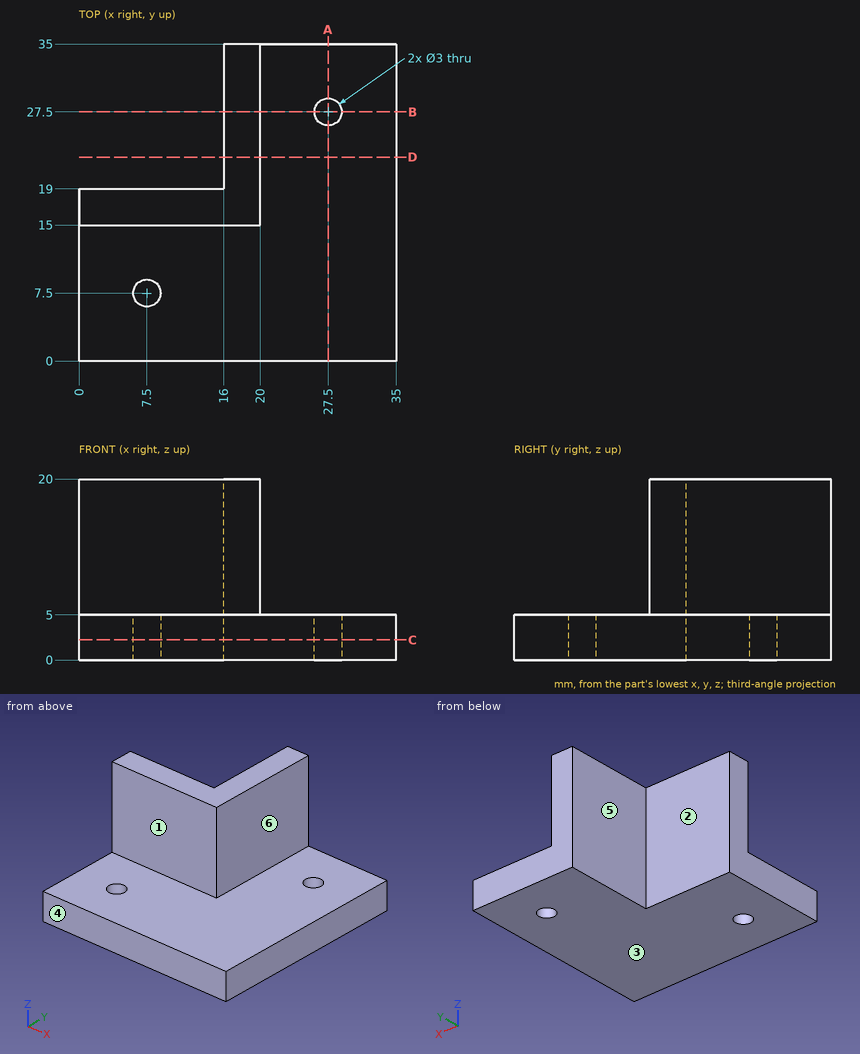
Study the drawing (mm; zero at the part's minimum x, y, z) and answer. A direction names the side the tool comes from. Coordinates: 2 decimals unless noted, no trailing zeros. Write each loop counter-clockwise with the first axis right and the second up, starting at its lowest first coordinate (ties: lowest second). Pieces come first, ordered by that corner, then holes. Notation, with made-up numbers: (85, 61.25) - (107, 61.25) arc R9 cw to (107, 78.25) - close; hole circle Ø11 at (32, 5). An arc over 180 degrees is marked (long way). One line per item, written item: value.
1) Find section A-A (x = 27.5). Give the vertices of the cut face in (y, z), and give its area (3 significant figures).
Geometry check:
outline: (0, 0) - (26, 0) - (26, 5) - (0, 5) - close; (29, 0) - (35, 0) - (35, 5) - (29, 5) - close
area: 160 mm2
2) Each of these flat-tipped pins is pushed along its axis until it touches: pin 1 Ø12 at (y, z) = (28.5, 16) entering from +X; pin 2 Ø5 at (y, z) = (25.5, 6.5) entering from -X; pin 3 Ø1.5 at (x, y) = (22.5, 15.5) entering from +Z. Where does it stop, or does it pass through?
Geometry check:
pin 1: stops at x = 20
pin 2: stops at x = 16
pin 3: stops at z = 5
3) A tool of negligible diameter and unlimited length cuts with its end or side. For the marked faces 4, 5 and 6, from which of +Z, -Z, +X, -X, +Y, -Y can it reach the whole face along a straight path? Write none if from no direction.
Geometry check:
face 4: +Z, -Z, +X, -X, -Y
face 5: +Z, -Z, -X, +Y
face 6: +Z, +X, +Y, -Y
4) For a pull along Y with two mould halves and no side action, classify the marked faces 1, 2 and 3 as pulls with the +Y half, pulls with the -Y half, needs draft (parallel to the pull), parting line crosses it, or undercut.
Geometry check:
face 1: pulls with the -Y half
face 2: pulls with the +Y half
face 3: needs draft
5) Find section D-D (y = 22.5). Give the vertices of the cut face in (x, z).
Geometry check:
outline: (16, 0) - (35, 0) - (35, 5) - (20, 5) - (20, 20) - (16, 20) - close
6) Find section B-B (y = 27.5). Give the vertices of the cut face in (x, z), and give its area (3 significant figures).
Geometry check:
outline: (16, 0) - (26, 0) - (26, 5) - (20, 5) - (20, 20) - (16, 20) - close; (29, 0) - (35, 0) - (35, 5) - (29, 5) - close
area: 140 mm2
7) Find section C-C (z = 2.25). Give the vertices of the cut face in (x, y).
Geometry check:
outline: (0, 0) - (35, 0) - (35, 35) - (16, 35) - (16, 19) - (0, 19) - close; hole circle Ø3 at (7.5, 7.5); hole circle Ø3 at (27.5, 27.5)
8) Consider line 1 along Y through (x, z) = (27.5, 1.1); line 2 along Y through (x, z) = (8, 14); line 3 along Z through (x, y) = (20, 5). Determine where each line is inside the solid, lowest interval first. Write a range as from..to.
Geometry check:
line 1: y = 0..26, 29..35
line 2: y = 15..19
line 3: z = 0..5
